Verification items for the finished model (mm, model axes). A direction names the side the tool comes from. Round coordinates to 2 decimals unless told otherwise and drop trailing zeros. Write each loop counter-clockwise with the first axis right and the second up, starting at its lowest first coordinate (ties: lowest second). Pieces come first, ordered by that corner, then holes. Notation, with made-up numbers: (8, 5.5) -> (50, 5.5) arc R26 cw to (50, 33.5) -> close; hole circle Ø9 at (40.5, -7.75). An arc over 180 degrees is marked (long way). Use CSV: the item, a comma, the result in double quotes.
Autodesk Inventor part; units mm, degrees
ref_plane "YZ Plane" through (0, 0, 0) normal (1, 0, 0) x (0, 1, 0)
ref_plane "XZ Plane" through (0, 0, 0) normal (0, 1, 0) x (-1, 0, 0)
ref_plane "XY Plane" through (0, 0, 0) normal (0, 0, 1) x (1, 0, 0)
sketch "Sketch1" plane through (0, 0, 0) normal (0, 1, 0) x (-1, 0, 0)
  line L0 (6.35, -3.6662) -> (0, -7.3323)
  line L1 (0, -7.3323) -> (-6.35, -3.6662)
  line L2 (-6.35, -3.6662) -> (-6.35, 3.6662)
  line L3 (-6.35, 3.6662) -> (0, 7.3323)
  line L4 (0, 7.3323) -> (6.35, 3.6662)
  line L5 (6.35, 3.6662) -> (6.35, -3.6662)
  point P0 (0, 0)
  point P1 (0, 0)
  point P2 (0, 0)
  dimension "d0" = 12.7
extrude "Extrusion1" add sketch "Sketch1" along normal blind 114.3
sketch "Sketch2" plane through (0, 0, 0) normal (0, -1, 0) x (1, 0, 0)
  point P0 (0, 0)
  point P1 (0, 0)
hole "Hole1" at (0, 0, 0) direction (0, 1, 0) diameter 4.9784 depth 25.4
sketch "Sketch3" plane through (0, 114.3, 0) normal (0, 1, 0) x (1, 0, 0)
  point P0 (0, 0)
  point P1 (0, 0)
hole "Hole2" at (0, 114.3, 0) direction (0, -1, 0) diameter 4.9784 depth 25.4
properties part number "SHOT_1_003_Hexshaft1" material "Aluminum 6061"
Q1. Material ranges on L1, parallel to Z at x = 0, y = 98.5; L2, parallel to X at y = 13.75, z = 0; L3, parallel to Z at x = -1.75, y = 24, recorded low to high.
Filled in:
L1,"-7.33 to -2.49, 2.49 to 7.33"
L2,"-6.35 to -2.49, 2.49 to 6.35"
L3,"-6.32 to -1.77, 1.77 to 6.32"
Q2. Section check D-D (x = 3.75). Record the cut outline in (y, z).
Filled in:
outline,"(0, -5.17) -> (114.3, -5.17) -> (114.3, 5.17) -> (0, 5.17) -> close"
Q3. Section check A-A (y = 14). Record the cut outline in (x, z), plus the area to 3 significant figures.
Filled in:
outline,"(-6.35, -3.67) -> (0, -7.33) -> (6.35, -3.67) -> (6.35, 3.67) -> (0, 7.33) -> (-6.35, 3.67) -> close; hole circle Ø4.98 at (0, 0)"
area,"120 mm²"
Q4. Section check C-C (y = 82). Record the cut outline in (x, z).
Filled in:
outline,"(-6.35, -3.67) -> (0, -7.33) -> (6.35, -3.67) -> (6.35, 3.67) -> (0, 7.33) -> (-6.35, 3.67) -> close"
Q5. Access from +Z, -Z, +X, -X, +Y, -Y to the whole of each face (thin tool, end or side, straight path). Record for faces 1 (the flat face through (0, 25.4, 0)), 2 (the flat face through (0, 88.9, 0)), 3 (the flat face through (3.219, 56.35, 5.474)).
Filled in:
face 1,"-Y"
face 2,"+Y"
face 3,"+Z, +X, +Y, -Y"
Q6. Section check B-B (z = 0). Record the cut outline in (x, y).
Filled in:
outline,"(-6.35, 0) -> (-2.49, 0) -> (-2.49, 25.4) -> (2.49, 25.4) -> (2.49, 0) -> (6.35, 0) -> (6.35, 114.3) -> (2.49, 114.3) -> (2.49, 88.9) -> (-2.49, 88.9) -> (-2.49, 114.3) -> (-6.35, 114.3) -> close"
Q7. Mould release check, pull along X, two halves, no side actions. Record for faces 4 (the flat face through (-3.131, 56.35, 5.525)), 5 (the cylindrical face through (-0.748, 12.878, -2.374)), 6 (the flat face through (3.131, 56.35, -5.525)), 7 (the cylindrical face through (-0.748, 101.422, 2.374)): released by +X, released by -X, zero draft, split by the parting line, or undercut.
Filled in:
face 4,"released by -X"
face 5,"undercut"
face 6,"released by +X"
face 7,"undercut"
Q8. Go/stop test with flat-tipped pins: P1, Ø8, axis at y = 59, z = 4.5, coming from the -X side; P2, Ø5, axis at x = -4, y = 13.5, coming from the +Z side; P3, Ø1.5, axis at x = -1, y = 31.5, coming from the -Z side; P4, Ø2.5, axis at x = -1, z = -0.5, coming from the +Y side. Record where each tip stops, or that it passes through.
Filled in:
P1,"x = -6.35"
P2,"z = 6.47"
P3,"z = -7.19"
P4,"y = 88.9"
